CAD build for the part. Positions are in the model's coordinates, mm. A direction names the side the tool comes from. Round coordinates to 2 decimals unless told otherwise and drop trailing zeros. Loops run counter-clockwise (first coordinate to the right, second up) from the corner with the lowest first, then second, coordinate; pieces in that order, holes last. Notation, with made-up numbers: (-10, -33.75) -> (38, -33.75) arc R4 cw to (38, -29.75) -> close; hole circle Ø9 at (1.25, 29). An arc over 180 degrees is marked (long way). Answer as CSV lines item,"result".
```python
from build123d import *

# Parameters (mm, degrees)
BOSS_EXTRUDE1_DEPTH = 2
BOSS_EXTRUDE2_START = 2
BOSS_EXTRUDE2_DEPTH = 2


with BuildPart() as part:
    # Sketch2 → Boss-Extrude1 (new body)
    with BuildSketch(Plane.XY.offset(4)):
        with BuildLine():
            Line((-44.305483114, -62), (-0.949182939, -62))
            ThreePointArc((-0.949182939, -62), (-0.521138453, -61.903757665), (-0.175485968, -61.633555836))
            ThreePointArc((-0.175485968, -61.633555836), (32.378563383, -27.679914383), (69.824948938, 0.787331812))
            ThreePointArc((69.824948938, 0.787331812), (70.23551024, 1.935299571), (69.231475595, 2.626895546))
            Line((69.231475595, 2.626895546), (0.749958934, -0.962068664))
            ThreePointArc((0.749958934, -0.962068664), (0.423121019, -1.035372755), (0.13882509, -1.212495134))
            ThreePointArc((0.13882509, -1.212495134), (-25.448078904, -26.366894393), (-48.317042245, -54.015474353))
            ThreePointArc((-48.317042245, -54.015474353), (-48.773291762, -59.244701736), (-44.305483114, -62))
        make_face()
        with BuildLine():
            Line((69.283811551, 1.628266012), (0.80229489, -1.960698198))
            ThreePointArc((0.80229489, -1.960698198), (-24.711294193, -27.043021815), (-47.514730419, -54.612379482))
            ThreePointArc((-47.514730419, -54.612379482), (-47.879730032, -58.795761389), (-44.305483114, -61))
            Line((-44.305483114, -61), (-0.949182939, -61))
            ThreePointArc((-0.949182939, -61), (31.7130194, -26.933555752), (69.283811551, 1.628266012))
        make_face(mode=Mode.SUBTRACT)
    extrude(amount=-BOSS_EXTRUDE1_DEPTH)

    # Sketch3 → Boss-Extrude2 (add)
    with BuildSketch(Plane.XY.offset(4).offset(BOSS_EXTRUDE2_START)):
        with BuildLine():
            Line((73.03813327, 2.826394022), (72.985797314, 3.825023556))
            Line((72.985797314, 3.825023556), (0.348531139, 0.018265743))
            ThreePointArc((0.348531139, 0.018265743), (0.022157357, -0.054848295), (-0.261851868, -0.231495595))
            ThreePointArc((-0.261851868, -0.231495595), (-26.066145165, -25.561463063), (-49.119354071, -53.418569223))
            ThreePointArc((-49.119354071, -53.418569223), (-49.666853492, -59.693642083), (-44.305483114, -63))
            Line((-44.305483114, -63), (-0.475074433, -63))
            Line((-0.475074433, -63), (-0.475074433, -62))
            ThreePointArc((-0.475074433, -62), (33.625159473, -26.574476321), (73.03813327, 2.826394022))
        make_face()
    extrude(amount=-BOSS_EXTRUDE2_DEPTH)


solid = part.part
```
Q1. Slice it at B-B, the plane x = -29. Give the cut face in (y, z).
Results:
outline,"(-63, 4) -> (-62, 4) -> (-62, 2) -> (-61, 2) -> (-61, 4) -> (-31.8, 4) -> (-31.8, 2) -> (-30.3, 2) -> (-30.3, 4) -> (-28.8, 4) -> (-28.8, 6) -> (-63, 6) -> close"
Q2. Drop flat-ended pins along their axis: pin 1 Ø10 at (x, y) = (17.5, -16) entering from -Z; pin 2 Ø1.6 at (x, z) = (-19.5, 3.5) entering from +Y; pin 3 Ø0.6 at (x, z) = (-26, 3) entering from -Y. Give the stop position or say it passes through.
Results:
pin 1,"z = 4"
pin 2,"y = -17.96"
pin 3,"y = -62"
Q3. Slice it at C-C, the plane y = -6.5. Give the cut face in (x, z), and give its area (3 significant figures).
Results:
outline,"(-7.16, 4) -> (-5.69, 4) -> (-5.69, 2) -> (-4.22, 2) -> (-4.22, 4) -> (57.29, 4) -> (57.29, 2) -> (59.02, 2) -> (59.02, 6) -> (-7.16, 6) -> close"
area,"139 mm2"
Q4. Tool access for faces 5 (the flat face through (19.1, -39.1, 2)), 6 (the cylindrical face through (-25.723, -25.189, 5.014)), 7 (the cylindrical face through (-25.11, -26, 3.01)), 8 (the cylindrical face through (-47.907, -58.74, 3.014)), 9 (the cylindrical face through (-48.807, -59.175, 3.014)): list every direction of +Z, -Z, +X, -X, +Y, -Y with a clear straight run to the whole face (end or side of a thin tool).
Results:
face 5,"-Z, +X, -X, +Y, -Y"
face 6,"+Z, -Z, -X, +Y"
face 7,"-Z, -X, +Y"
face 8,"-Z"
face 9,"-Z, -X"
Q5. Probe L1, parallel to Z at x = 29, y = -10.5; L2, parallel to Y at x = 55, z = 3.75; L3, parallel to X at y = -10.5, z = 3.9. List the from-to ranges inside material, lowest first. Write a range as [from, to].
Results:
L1,"[4, 6]"
L2,"[-9.39, -8.15], [0.88, 1.88]"
L3,"[-9.93, -8.48], [51.82, 53.49]"
Q6. Slice it at D-D, the plane y = -45.5. Give the cut face in (x, z), and give its area (3 significant figures).
Results:
outline,"(-43.05, 4) -> (-41.78, 4) -> (-41.78, 2) -> (-40.5, 2) -> (-40.5, 4) -> (12.65, 4) -> (12.65, 2) -> (14.03, 2) -> (14.03, 6) -> (-43.05, 6) -> close"
area,"119 mm2"
Q7. Slice it at A-A, the plane z = 2.85. Give the cut face in (x, y).
Results:
outline,"(-48.32, -54.02) arc R5 ccw to (-44.31, -62) -> (-0.95, -62) arc R1 ccw to (-0.18, -61.63) arc R301 cw to (69.82, 0.79) arc R1 ccw to (69.23, 2.63) -> (0.75, -0.96) arc R1 ccw to (0.14, -1.21) arc R349 ccw to start; hole (-47.51, -54.61) arc R4 ccw to (-44.31, -61) -> (-0.95, -61) arc R302 cw to (69.28, 1.63) -> (0.8, -1.96) arc R348 ccw to start"
Q8. Two-plate mould, pull along Y, no slides. Class faces 1 (the cylindrical face through (-24.37, -26.67, 3.01)), 2 (the flat face through (35.47, 0.858, 3.014)), 3 (the flat face through (16, 0, 4)), 4 (the cylindrical face through (-49.71, -59.61, 5.01)): pulls with the +Y half, pulls with the -Y half, needs draft (parallel to the pull), parting line crosses it, or undercut.
Results:
face 1,"undercut"
face 2,"pulls with the +Y half"
face 3,"needs draft"
face 4,"parting line crosses it"
